from build123d import *

# Parameters (mm, degrees)
SKETCH1_R           = 10.5
BOSS_EXTRUDE1_DEPTH = 12
CUT_EXTRUDE1_DEPTH  = 13
BOSS_EXTRUDE2_DEPTH = 12
CUT_EXTRUDE2_DEPTH  = 13
SKETCH5_R           = 2.75
CUT_EXTRUDE3_DEPTH  = 11
SKETCH7_R           = 12
CUT_EXTRUDE4_DEPTH  = 10
SKETCH10_W          = 18
SKETCH10_H          = 1
CUT_EXTRUDE5_DEPTH  = 13
SKETCH11_W          = 1.35
SKETCH11_H          = 0.6


with BuildPart() as part:
    # Sketch1 → Boss-Extrude1 (new body)
    with BuildSketch(Plane.XY):
        Polygon((-28, -40), (28, -40), (28, -30), (16, -30), (16, 16), (-16, 16), (-16, -30), (-28, -30), align=None)
        Circle(SKETCH1_R, mode=Mode.SUBTRACT)
    extrude(amount=BOSS_EXTRUDE1_DEPTH)

    # Sketch2 → Cut-Extrude1 (cut, through all)
    with BuildSketch(Plane.XY):
        with BuildLine():
            Line((3, 16), (16, 16))
            Line((16, 16), (16, 3))
            ThreePointArc((16, 3), (12.192388155, 12.192388155), (3, 16))
        make_face()
        with BuildLine():
            Line((-3, 16), (-16, 16))
            Line((-16, 16), (-16, 3))
            ThreePointArc((-16, 3), (-12.192388155, 12.192388155), (-3, 16))
        make_face()
    extrude(amount=CUT_EXTRUDE1_DEPTH, mode=Mode.SUBTRACT)

    # Sketch3 → Boss-Extrude2 (add, through all)
    with BuildSketch(Plane.XY):
        with BuildLine():
            Line((16, -29.5), (16, -30))
            Line((16, -30), (16.5, -30))
            ThreePointArc((16.5, -30), (16.146446609, -29.853553391), (16, -29.5))
        make_face()
        with BuildLine():
            Line((-16, -29.5), (-16, -30))
            Line((-16, -30), (-16.5, -30))
            ThreePointArc((-16.5, -30), (-16.146446609, -29.853553391), (-16, -29.5))
        make_face()
    extrude(amount=BOSS_EXTRUDE2_DEPTH)

    # Sketch4 → Cut-Extrude2 (cut, through all)
    with BuildSketch(Plane.XY):
        with BuildLine():
            Line((-27.5, -30), (-28, -30))
            Line((-28, -30), (-28, -30.5))
            ThreePointArc((-28, -30.5), (-27.853553391, -30.146446609), (-27.5, -30))
        make_face()
        with BuildLine():
            Line((27.5, -30), (28, -30))
            Line((28, -30), (28, -30.5))
            ThreePointArc((28, -30.5), (27.853553391, -30.146446609), (27.5, -30))
        make_face()
    extrude(amount=CUT_EXTRUDE2_DEPTH, mode=Mode.SUBTRACT)

    # Sketch5 → Cut-Extrude3 (cut, through all)
    with BuildSketch(Plane(origin=(0, -30, 0), x_dir=(1, 0, 0), z_dir=(0, 1, 0))):
        with Locations((-22, -6)):
            Circle(SKETCH5_R)
        with Locations((22, -6)):
            Circle(SKETCH5_R)
    extrude(amount=-CUT_EXTRUDE3_DEPTH, mode=Mode.SUBTRACT)

    # Sketch7 → Cut-Extrude4 (cut)
    with BuildSketch(Plane.XY.offset(12)):
        Circle(SKETCH7_R)
    extrude(amount=-CUT_EXTRUDE4_DEPTH, mode=Mode.SUBTRACT)

    # Sketch10 → Cut-Extrude5 (cut, through all)
    with BuildSketch(Plane.XY.offset(12)):
        with Locations((0, -39.5)):
            Rectangle(SKETCH10_W, SKETCH10_H)
    extrude(amount=-CUT_EXTRUDE5_DEPTH, mode=Mode.SUBTRACT)

    # Sketch11 → Cut-Revolve1 (revolve, cut)
    with BuildSketch(Plane(origin=(0, 0, 0), x_dir=(0, 0, -1), z_dir=(1, 0, 0))):
        with Locations((-8.525, 12.3)):
            Rectangle(SKETCH11_W, SKETCH11_H)
    revolve(axis=Axis((0, 0, -88.99), (0, 0, 1)), mode=Mode.SUBTRACT)


solid = part.part
The model under review builds one solid part; all positions refer to its coordinate system, in mm. A direction names the side the tool comes from. Coordinates: 2 decimals unless noted, no trailing zeros. Loops run counter-clockwise (first coordinate to the right, second up) from the corner with the lowest first, then second, coordinate; pieces in that order, holes last.
(1) Consider section A-A, the plane y = 0. Give the boundary of the cut face in (x, z), plus the area to 3 significant figures.
Determined:
outline: (-16, 0) - (-10.5, 0) - (-10.5, 2) - (-12, 2) - (-12, 7.85) - (-12.6, 7.85) - (-12.6, 9.2) - (-12, 9.2) - (-12, 12) - (-16, 12) - close; (10.5, 0) - (16, 0) - (16, 12) - (12, 12) - (12, 9.2) - (12.6, 9.2) - (12.6, 7.85) - (12, 7.85) - (12, 2) - (10.5, 2) - close
area: 100 mm2
(2) Insertion check: P1, Ø6, axis at y = 9.5, z = 1.5, coming from the -X side; P2, Ø3.5, axis at y = -20, z = 6, coming from the -X side; P3, Ø12, axis at x = -2.5, y = 4, coming from the +Z side. Each pin has a flat end and moves straight along its axis. Give the tip position at first contact, or say it passes through.
Determined:
P1: stops at x = -15.52
P2: stops at x = -16
P3: stops at z = 2
(3) Consider section C-C, the plane x = -22. Give the boundary of the cut face in (y, z).
Determined:
outline: (-40, 0) - (-30, 0) - (-30, 3.25) - (-40, 3.25) - close; (-40, 8.75) - (-30, 8.75) - (-30, 12) - (-40, 12) - close
(4) Consider section D-D, the plane y = -19. Give the boundary of the cut face in (x, z).
Determined:
outline: (-16, 0) - (16, 0) - (16, 12) - (-16, 12) - close
(5) Consider section B-B, the plane z = 6. Give the boundary of the cut face in (x, y).
Determined:
outline: (-28, -40) - (-24.75, -40) - (-24.75, -30) - (-27.5, -30) arc R0.5 ccw to (-28, -30.5) - close; (-19.25, -40) - (-9, -40) - (-9, -39) - (9, -39) - (9, -40) - (19.25, -40) - (19.25, -30) - (16.5, -30) arc R0.5 cw to (16, -29.5) - (16, 3) arc R13 ccw to (3, 16) - (-3, 16) arc R13 ccw to (-16, 3) - (-16, -29.5) arc R0.5 cw to (-16.5, -30) - (-19.25, -30) - close; (24.75, -40) - (28, -40) - (28, -30.5) arc R0.5 ccw to (27.5, -30) - (24.75, -30) - close; hole circle Ø24 at (0, 0)
(6) Draft analysis for pull direction Y (two halves, no side actions). For faces 5 (the flat face through (28, -35, 6)), 6 (the flat face through (0, -11, 2)), 7 (the flat face through (0, 16, 6)), 8 (the flat face through (-19, -40, 6)), state which applies: +Y half, -Y half, draft (parallel to the pull), parting line (faces both ways), or undercut.
Determined:
face 5: draft
face 6: undercut
face 7: +Y half
face 8: -Y half
(7) Tool access review of faces 1 (the flat face through (22, -30, 3)), 2 (the cylindrical face through (-3.78, 12.02, 8.52)), 3 (the flat face through (-22, -30, 3)), 4 (the cylindrical face through (11.446, 3.604, 4.966)): name each direction out of +Z, -Z, +X, -X, +Y, -Y from which nothing blocks a thin tool from reaching the whole face with its end or side.
Determined:
face 1: +Z, -Z, +X, +Y
face 2: none
face 3: +Z, -Z, -X, +Y
face 4: +Z
(8) Wall thickness on L1, parallel to Z at x = 22, y = -37; L2, parallel to X at y = -33.5, z = 4.75; L3, parallel to X at y = 0, z = 8.5: over which ranges is each line inside the solid? List them lowest first.
Determined:
L1: z = 0 to 3.25, 8.75 to 12
L2: x = -28 to -24.45, -19.55 to 19.55, 24.45 to 28
L3: x = -16 to -12.6, 12.6 to 16
